```python
from build123d import *

# Parameters (mm, degrees)
SKETCH1_R           = 52
BOSS_EXTRUDE1_DEPTH = 165
BOSS_EXTRUDE2_DEPTH = 5
LPATTERN1_COUNT     = 7
LPATTERN1_PITCH     = 20
BOSS_EXTRUDE3_DEPTH = 12
SKETCH4_R           = 47
CUT_EXTRUDE1_DEPTH  = 172


with BuildPart() as part:
    # Sketch1 → Boss-Extrude1 (new body)
    with BuildSketch(Plane(origin=(0, 0, 0), x_dir=(1, 0, 0), z_dir=(0, 1, 0))):
        with Locations(Location((0, 0, 0), (0, 0, 270))):
            Circle(SKETCH1_R)
    extrude(amount=-BOSS_EXTRUDE1_DEPTH)

    # Sketch2 → Boss-Extrude2 (add)
    with BuildSketch(Plane(origin=(0, 0, 0), x_dir=(1, 0, 0), z_dir=(0, 1, 0))):
        with BuildLine():
            Line((-44, -60), (44, -60))
            ThreePointArc((44, -60), (61.67766953, -52.67766953), (69, -35))
            Line((69, -35), (69, 35))
            ThreePointArc((69, 35), (61.67766953, 52.67766953), (44, 60))
            Line((44, 60), (-44, 60))
            ThreePointArc((-44, 60), (-61.67766953, 52.67766953), (-69, 35))
            Line((-69, 35), (-69, -35))
            ThreePointArc((-69, -35), (-61.67766953, -52.67766953), (-44, -60))
        make_face()
    boss_extrude2 = extrude(amount=-BOSS_EXTRUDE2_DEPTH)

    # LPattern1: Boss-Extrude2 ×7
    with Locations(*[(0, -i * LPATTERN1_PITCH, 0) for i in range(1, LPATTERN1_COUNT)]):
        add(boss_extrude2)

    # Sketch3 → Boss-Extrude3 (add)
    with BuildSketch(Plane.XZ.offset(165)):
        Polygon((-43, 55), (-58, 40), (-58, -40), (-43, -55), (43, -55), (58, -40), (58, 40), (43, 55), align=None)
    extrude(amount=BOSS_EXTRUDE3_DEPTH)

    # Sketch4 → Cut-Extrude1 (cut)
    with BuildSketch(Plane.XZ.offset(177)):
        with Locations(Location((0, 0, 0), (0, 0, 270))):
            Circle(SKETCH4_R)
    extrude(amount=-CUT_EXTRUDE1_DEPTH, mode=Mode.SUBTRACT)


solid = part.part
```
For this review, take the finished solid that the model builds, in its own axes (mm). A direction names the side the tool comes from. Round coordinates to 2 decimals unless told otherwise and drop trailing zeros. Order: outer loops, then holes, each group sorted by start corner. A loop starts at its lowest first (then second) coordinate and runs counter-clockwise, first axis right, second up.
Q1. Mouldability with a two-part tool opening along Y and no side actions: class faces 3 (the cylindrical face through (-31.641, -32.395, -41.265)), 4 (the flat face through (-1, 0, -1)), 5 (the flat face through (69, -62, 0)) as pulls with the +Y half, pulls with the -Y half, needs draft (parallel to the pull), parting line crosses it, or undercut.
Findings below:
face 3: undercut
face 4: pulls with the +Y half
face 5: needs draft
Q2. Wall thickness on line 1 (X direction, y = -141.5, z = 0); line 2 (Y direction, x = -38.5, z = -19); line 3 (Z direction, x = -31, y = -107): over which ranges is each line inside the solid? List them lowest first.
Findings below:
line 1: x = -52 to -47, 47 to 52
line 2: y = -5 to 0
line 3: z = -41.75 to -35.33, 35.33 to 41.75
Q3. Insertion check: P1, Ø12, axis at y = -32, z = 3.5, coming from the +X side; P2, Ø6, axis at x = -11, z = -47, coming from the +Y side; P3, Ø1, axis at x = -27, y = -138, coming from the +Z side; P4, Ø8, axis at x = 20.5, z = -34.5, coming from the -Y side. Each pin has a flat end and moves straight along its axis. Give the tip position at first contact, or say it passes through.
Findings below:
P1: stops at x = 52
P2: stops at y = 0
P3: stops at z = 44.74
P4: stops at y = -5
Q4. We need section A-A, the plane y = -31. Give the boundary of the cut face in (x, z).
Findings below:
outline: circle Ø104 at (0, 0); hole circle Ø94 at (0, 0)
Q5. Machinability: for faces 1 (the cylindrical face through (61.871, -82.465, -52.482)), 2 (the cylindrical face through (-31.641, -72.395, -41.265)), which of the approach directions +Z, -Z, +X, -X, +Y, -Y give a long, thin tool a straight path to every point of the face, cutting with its end or side? Answer none if there is none.
Findings below:
face 1: -Z, +X, +Y, -Y
face 2: none
